Design review of the part built by this model. Coordinates are the model's own, in mm. Face numbers are marked on the shaded views. A direction names the side the tool comes from. Give positions to 0.01 mm unless a question says otherwise; leave off trailing zeros. Write each loop counter-clockwise with the first axis right and the second up, starting at its lowest first coordinate (ties: lowest second). Pieces come first, ordered by that corner, then holes. Notation, with made-up numbers: M 71.25,89 L 124.25,89 A22 ccw 124.25,117 Z; hole C 43,-29 d7. An arc over 180 degrees is marked long. Use a Markdown table: item, result. Add a question column.
```python
from build123d import *

# Parameters (mm, degrees)
F0_W      = 39
F0_H      = 39
F1_DEPTH  = 13
F3_R      = 3.25
F5_DEPTH  = 11
F2_R      = 1.8
F2_W      = 17
F2_H      = 8
F6_DEPTH  = 13.001
F7_R      = 1.5
F12_W     = 7.1
F12_H     = 4.5
F13_DEPTH = 0.97705
F14_W     = 13.5
F14_H     = 4.5
F15_DEPTH = 0.97705


with BuildPart() as f1:
    # F0 (on Top) → F1 (new body)
    with BuildSketch(Plane.XY):
        Rectangle(F0_W, F0_H)
    extrude(amount=-F1_DEPTH)

    # F3
    f3_edges = [f1.edges().sort_by_distance(p)[0] for p in [
        (-19.5, -19.5, -6.5),
        (19.5, -19.5, -6.5),
        (19.5, 19.5, -6.5),
        (-19.5, 19.5, -6.5),
    ]]
    fillet(f3_edges, radius=F3_R)

    # F4 (on Top) → F5 (cut)
    with BuildSketch(Plane.XY):
        with BuildLine():
            ThreePointArc((-18.52295, -15.27295), (-17.571047, -17.571047), (-15.27295, -18.52295))
            Line((-15.27295, -18.52295), (15.27295, -18.52295))
            ThreePointArc((15.27295, -18.52295), (17.571047, -17.571047), (18.52295, -15.27295))
            Line((18.52295, -15.27295), (18.52295, 15.27295))
            ThreePointArc((18.52295, 15.27295), (17.571047, 17.571047), (15.27295, 18.52295))
            Line((15.27295, 18.52295), (-15.27295, 18.52295))
            ThreePointArc((-15.27295, 18.52295), (-17.571047, 17.571047), (-18.52295, 15.27295))
            Line((-18.52295, 15.27295), (-18.52295, -15.27295))
        make_face()
    extrude(amount=-F5_DEPTH, mode=Mode.SUBTRACT)

    # F2 (on face) → F6 (cut, through all)
    with BuildSketch(Plane(origin=(0, 0, -13), x_dir=(1, 0, 0), z_dir=(0, 0, -1))):
        with Locations((-15.25, 15.25)):
            Circle(F2_R)
        with Locations((15.25, 15.25)):
            Circle(F2_R)
        with Locations((-15.25, -15.25)):
            Circle(F2_R)
        with Locations((15.25, -15.25)):
            Circle(F2_R)
        with Locations((2.75, -13.25)):
            Rectangle(F2_W, F2_H)
    extrude(amount=-F6_DEPTH, mode=Mode.SUBTRACT)

    # F7
    f7_edges = [f1.edges().sort_by_distance(p)[0] for p in [
        (0, -19.5, -13),
    ]]
    fillet(f7_edges, radius=F7_R)

    # F12 (on face) → F13 (cut, through all)
    with BuildSketch(Plane(origin=(-19.5, 0, 0), x_dir=(0, -1, 0), z_dir=(-1, 0, 0))):
        with Locations((6.7, -2.25)):
            Rectangle(F12_W, F12_H)
        with Locations((-6.7, -2.25)):
            Rectangle(F12_W, F12_H)
    extrude(amount=-F13_DEPTH, mode=Mode.SUBTRACT)

    # F14 (on face) → F15 (cut, through all)
    with BuildSketch(Plane.XZ.offset(19.5)):
        with Locations((0, -2.25)):
            Rectangle(F14_W, F14_H)
    extrude(amount=-F15_DEPTH, mode=Mode.SUBTRACT)


solid = f1.part
```
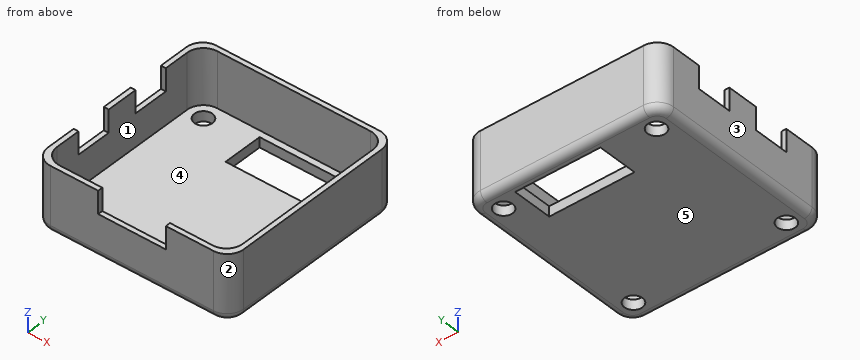
(1) Machinability: for the marked faces 1 and 2, which of the approach directions +Z, -Z, +X, -X, +Y, -Y give a long, thin tool a straight path to every point of the face, cutting with its end or side? Answer none if there is none.
(2) Add section C-C on x = 3.5. Give the boundary of the cut face in (y, z).
(3) Add section A-A on y = 11. Give the boundary of the cut face in (x, z).
(4) Add section B-B on z = -2. Give the boundary of the cut face in (x, y), then the cut area to 3 significant figures.
(5) For pin 1 (0.5 mm diameter, centred on y = -19, z = -1.5, fed in from +X); pin 2 (1.6 mm diameter, centred on y = 12.5, z = -12.5, fed in from +X); pin 3 (0.8 mm diameter, centred on x = -19, z = -2, fed in from +Y) (3 decimals), all flat-tipped, find the tip position at first contact; note any pin that passes through.
(6) Add section D-D on z = -7.5. Give the boundary of the cut face in (x, y), then the cut area to 3 significant figures.
(7) The part is to be moulded in two halves that separate along X. For the marked faces 3, 4 and 5, say which applies: released by +X, released by -X, zero draft, split by the parting line, or undercut.
(8) Wall thickness on L1, parallel to Y at x = -15.25, z = -11.55; L2, parallel to X at y = 15.25, z = -11.4: over which ranges is each line inside the solid? List them lowest first.
From the geometry:
| question | item | result |
|---|---|---|
| 1 | face 1 | +Z |
| 1 | face 2 | +Z, -Z, +X, -Y |
| 2 | outline | M -19.5,-11.5 A1.5 ccw -18,-13 L 9.25,-13 L 9.25,-11 L -18.52,-11 L -18.52,-4.5 L -19.5,-4.5 Z; M 17.25,-13 L 18,-13 A1.5 ccw 19.5,-11.5 L 19.5,0 L 18.52,0 L 18.52,-11 L 17.25,-11 Z |
| 3 | outline | M -19.5,-11.5 A1.5 ccw -18,-13 L -5.75,-13 L -5.75,-11 L -18.52,-11 L -18.52,0 L -19.5,0 Z; M 11.25,-13 L 18,-13 A1.5 ccw 19.5,-11.5 L 19.5,0 L 18.52,0 L 18.52,-11 L 11.25,-11 Z |
| 4 | outline | M -19.5,-16.25 A3.25 ccw -16.25,-19.5 L -6.75,-19.5 L -6.75,-18.52 L -15.27,-18.52 A3.25 cw -18.52,-15.27 L -18.52,-10.25 L -19.5,-10.25 Z; M -19.5,-3.15 L -18.52,-3.15 L -18.52,3.15 L -19.5,3.15 Z; M -19.5,10.25 L -18.52,10.25 L -18.52,15.27 A3.25 cw -15.27,18.52 L 15.27,18.52 A3.25 cw 18.52,15.27 L 18.52,-15.27 A3.25 cw 15.27,-18.52 L 6.75,-18.52 L 6.75,-19.5 L 16.25,-19.5 A3.25 ccw 19.5,-16.25 L 19.5,16.25 A3.25 ccw 16.25,19.5 L -16.25,19.5 A3.25 ccw -19.5,16.25 Z |
| 4 | area | 122 mm^2 |
| 5 | pin 1 | stops at x = 18.33 |
| 5 | pin 2 | stops at x = 19.49 |
| 5 | pin 3 | stops at y = 18.495 |
| 6 | outline | M -19.5,-16.25 A3.25 ccw -16.25,-19.5 L 16.25,-19.5 A3.25 ccw 19.5,-16.25 L 19.5,16.25 A3.25 ccw 16.25,19.5 L -16.25,19.5 A3.25 ccw -19.5,16.25 Z; hole M -18.52,-15.27 A3.25 ccw -15.27,-18.52 L 15.27,-18.52 A3.25 ccw 18.52,-15.27 L 18.52,15.27 A3.25 ccw 15.27,18.52 L -15.27,18.52 A3.25 ccw -18.52,15.27 Z |
| 6 | area | 149 mm^2 |
| 7 | face 3 | released by -X |
| 7 | face 4 | undercut |
| 7 | face 5 | zero draft |
| 8 | L1 | y = -19.5 to -17.05, -13.45 to 13.45, 17.05 to 19.5 |
| 8 | L2 | x = -19.5 to -17.05, -13.45 to -5.75, 11.25 to 13.45, 17.05 to 19.5 |
